Design review of the part built by this model. Coordinates are the model's own, in mm. Round coordinates to 2 decimals unless told otherwise and drop trailing zeros. Write each loop counter-clockwise with the first axis right and the second up, starting at its lowest first coordinate (ties: lowest second). Pieces come first, ordered by that corner, then holes. Notation, with made-up numbers: (67, 78.5) - (112, 78.5) arc R6 cw to (112, 86.5) - close; hole circle Ø9 at (72, 85.5). An arc over 180 degrees is marked (long way). Use one line per item in the form item = value.
```python
from build123d import *

# Parameters (mm, degrees)
SKETCH1_R           = 25
BOSS_EXTRUDE1_DEPTH = 2
SKETCH2_R           = 1
BOSS_EXTRUDE2_DEPTH = 1


with BuildPart() as part:
    # Sketch1 → Boss-Extrude1 (new body)
    with BuildSketch(Plane(origin=(0, 0, 0), x_dir=(1, 0, 0), z_dir=(0, 1, 0))):
        Circle(SKETCH1_R)
    extrude(amount=BOSS_EXTRUDE1_DEPTH)

    # Sketch2 → Boss-Extrude2 (add)
    with BuildSketch(Plane(origin=(0, 2, 0), x_dir=(1, 0, 0), z_dir=(0, 1, 0))):
        with Locations((0, 23)):
            Circle(SKETCH2_R)
        with Locations((23, 0)):
            Circle(SKETCH2_R)
        with Locations((0, -23)):
            Circle(SKETCH2_R)
        with Locations((-23, 0)):
            Circle(SKETCH2_R)
    extrude(amount=BOSS_EXTRUDE2_DEPTH)


solid = part.part
```
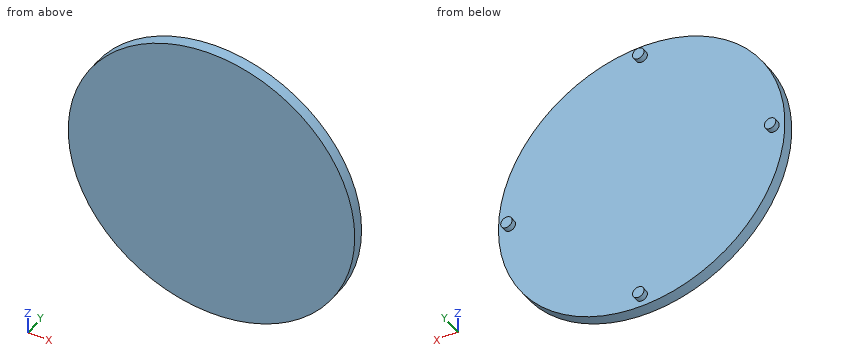
Q1. For P1, Ø1.5, axis at x = -11.5, z = 19, coming from the +Y side; P2, Ø1.5, axis at y = 2, z = -18, coming from the -X side; P3, Ø1, axis at x = 1.5, y = 1, coming from the +Z side, all flat-tipped, find the tip position at first contact; note any pin that passes through.
Calculated:
P1 = 2
P2 = -18.1
P3 = 24.98
Q2. We need section C-C on z = -15. Write out the cut boundary in (x, y), then the cut area to 3 significant figures.
Calculated:
outline = (-20, 0) - (20, 0) - (20, 2) - (-20, 2) - close
area = 80.0 mm2
Q3. We need section A-A on x = 0. Write out the cut boundary in (y, z), then the cut area to 3 significant figures.
Calculated:
outline = (0, -25) - (2, -25) - (2, -24) - (3, -24) - (3, -22) - (2, -22) - (2, 22) - (3, 22) - (3, 24) - (2, 24) - (2, 25) - (0, 25) - close
area = 104 mm2
Q4. We need section D-D on z = 23. Write out the cut boundary in (x, y).
Calculated:
outline = (-9.8, 0) - (9.8, 0) - (9.8, 2) - (1, 2) - (1, 3) - (-1, 3) - (-1, 2) - (-9.8, 2) - close
Q5. To check wall thickness, follow line 1 along X through (y, z) = (2.8, -0.5); line 2 along Y through (x, z) = (-17.5, -9); line 3 along X through (y, z) = (1.6, 4.5). State the ranges of each line that lie inside material, in increasing order. Write a range as from..to.
Calculated:
line_1 = -23.87..-22.13, 22.13..23.87
line_2 = 0..2
line_3 = -24.59..24.59
Q6. We need section B-B on y = 2.5. Write out the cut boundary in (x, z).
Calculated:
outline = circle Ø2 at (-23, 0); circle Ø2 at (0, -23); circle Ø2 at (0, 23); circle Ø2 at (23, 0)
